from build123d import *

# Parameters (mm, degrees)
BOX991_W           = 148
BOX991_H           = 40
BOX991_DEPTH       = 40
CYLINDER2098_R     = 16
CYLINDER2098_DEPTH = 6
CHAMFER080_SIZE    = 2


with BuildPart() as krychle991:
    # Box991 → Box991 (new body)
    with BuildSketch(Plane(origin=(-74, 42, 16), x_dir=(1, 0, 0), z_dir=(0, 0, 1))):
        with Locations((74, 20)):
            Rectangle(BOX991_W, BOX991_H)
    extrude(amount=BOX991_DEPTH)


with BuildPart() as chamfer080:
    # Cylinder2098 → Cylinder2098 (new body)
    with BuildSketch(Plane(origin=(0, 86, 16), x_dir=(1, 0, 0), z_dir=(0, 0, 1))):
        Circle(CYLINDER2098_R)
    extrude(amount=CYLINDER2098_DEPTH)

    # Cut691: cut Krychle991
    add(krychle991.part, mode=Mode.SUBTRACT)

    # Chamfer080
    chamfer080_edges = [chamfer080.edges().sort_by_distance(p)[0] for p in [
        (-2.016069, 101.872475, 16),
    ]]
    chamfer(chamfer080_edges, length=CHAMFER080_SIZE)


solid = chamfer080.part
Verification items for the finished model (mm, model axes). Give positions to 0.01 mm unless a question says otherwise; leave off trailing zeros. Loops run counter-clockwise (first coordinate to the right, second up) from the corner with the lowest first, then second, coordinate; pieces in that order, holes last. Notation, with made-up numbers: (64.5, -27.75) - (82.5, -27.75) arc R16 cw to (82.5, 0.25) - close; hole circle Ø6 at (0.25, 50). An arc over 180 degrees is marked (long way). Write each question's results on one line, items separated by ' | '.
1) Depth check by flat-ended pin: P1, Ø3, axis at x = 2, z = 18, coming from the +Y side. Enter the tip coordinate at first touch or a pass-through.
Solution:
P1: y = 101.99
2) Sectioned sample at C-C on z = 18.75. Record the boundary of the cut face in (x, y).
Solution:
outline: (-15.49, 82) - (15.49, 82) arc R16 ccw (long way) to start
3) Sectioned sample at D-D on z = 17. Record the boundary of the cut face in (x, y).
Solution:
outline: (-14.46, 82) - (14.46, 82) arc R15 ccw (long way) to start
4) Material ranges on L1, parallel to X at y = 90, z = 21.25; L2, parallel to X at y = 86.25, z = 18.5; L3, parallel to Y at x = -12.5, z = 21.5, recorded low to high. Write a range as from..to.
Solution:
L1: -15.49..15.49 | L2: -16..16 | L3: 82..95.99
5) Sectioned sample at B-B on y = 86. Record the boundary of the cut face in (x, z).
Solution:
outline: (-16, 18) - (-14, 16) - (14, 16) - (16, 18) - (16, 22) - (-16, 22) - close
6) Sectioned sample at A-A on x = 0. Record the boundary of the cut face in (y, z), plus the area to 3 significant figures.
Solution:
outline: (82, 16) - (100, 16) - (102, 18) - (102, 22) - (82, 22) - close | area: 118 mm2
